Input: dimensioned drawing with shaded views. Units: mm. Origin: part minimum x, y, z. A direction names the side the tool comes from. Give positions to 0.01 mm unless a question says otherwise; leave off trailing zeros. Loops run counter-clockwise (first coordinate to the right, second up) from the corner with the lowest first, then second, coordinate; pieces in that order, holes last. Notation, with made-up numbers: M 26,-39.75 L 32,-39.75 A23 cw 32,-7.75 Z; hole C 5,52.5 d4. An arc over 180 degrees is marked long. Answer in a Markdown table with one row per item.
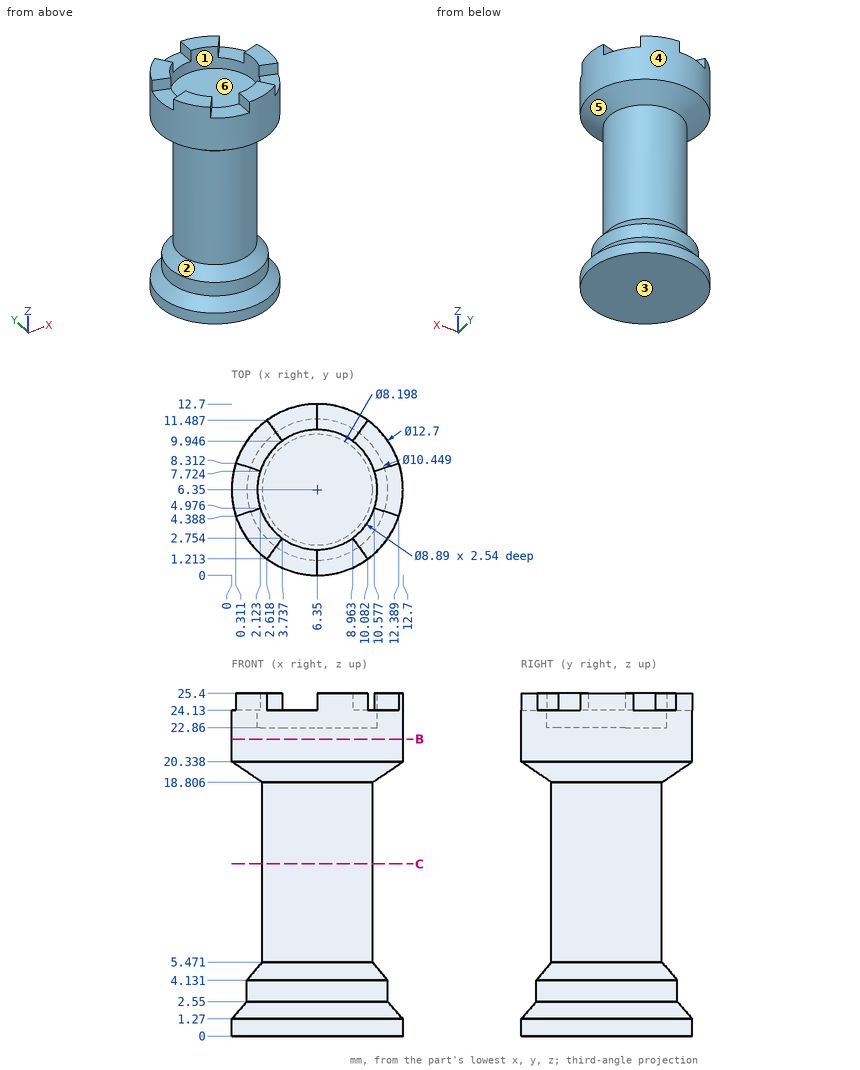
Q1. Contact query for flat-ended pins moving along their axis: pin 1 Ø5 at (y, z) = (5.5, 13) entering from -X; pin 2 Ø1.7 at (x, y) = (11, 9) entering from +Z; pin 3 Ø1.5 at (y, z) = (2, 18) entering from +X. Output: stop coordinate, or through.
Values follow:
| item | result |
|---|---|
| pin 1 | x = 2.25 |
| pin 2 | z = 24.13 |
| pin 3 | x = 8.31 |
Q2. Ray query, probe 1 along Y at (x, z) = (6.35, 23.55) (1 decimal); probe 2 along Z at (x, y) = (8.25, 4.5); probe 3 along Y at (x, z) = (9.5, 23.5) (1 decimal). Return the intervals inside material, ascending. Write a range as from..to.
Values follow:
| item | result |
|---|---|
| probe 1 | 0..1.9, 10.8..12.7 |
| probe 2 | 0..22.86 |
| probe 3 | 0.8..3.2, 9.5..11.9 |
Q3. Reachability of the marked faces 4, 5 and 6 from +Z, -Z, +X, -X, +Y, -Y: full face, straight path, thin tool, end or side. Return the list, or none.
Values follow:
| item | result |
|---|---|
| face 4 | +Z, -Z |
| face 5 | none |
| face 6 | +Z |
Q4. Section query B-B (z = 22). Output: boundary loops of the cut face in (x, y), plus the area to 3 significant figures.
Values follow:
| item | result |
|---|---|
| outline | C 6.35,6.35 d12.7 |
| area | 127 mm^2 |
Q5. Mould query, pull axis Z, two halves, no side actions, for the marked faces 1, 2 and 3. Classes: +Z half, -Z half, draft (parallel to the pull), parting line (faces both ways), or undercut.
Values follow:
| item | result |
|---|---|
| face 1 | draft |
| face 2 | undercut |
| face 3 | -Z half |
Q6. Section query C-C (z = 12.75). Output: boundary loops of the cut face in (x, y).
Values follow:
| item | result |
|---|---|
| outline | C 6.35,6.35 d8.2 |
